Model file for the job. Use its own axes, mm. Give positions to 0.01 mm unless a question says otherwise; leave off trailing zeros. Loops run counter-clockwise (first coordinate to the right, second up) from the corner with the lowest first, then second, coordinate; pieces in that order, holes last. Notation, with made-up numbers: M 17.5,0 L 49.5,0 A22 cw 49.5,29 Z; hole C 74.25,-40 d5. An arc over 180 degrees is marked long. Answer in a Markdown table with one row per item.
```python
from build123d import *

# Parameters (mm, degrees)
SKETCH2_W                            = 300
SKETCH2_H                            = 150
BOSS_EXTRUDE1_DEPTH                  = 1.52
F_4_0_4_DIAMETER_HOLE1_D             = 4
MIRROR1_AT_THE_SECOND_PLANE_COPY_1_D = 4
F_11_0_11_DIAMETER_HOLE4_D           = 11
F_11_0_11_DIAMETER_HOLE2_D           = 11
F_11_0_11_DIAMETER_HOLE3_D           = 11


with BuildPart() as part:
    # Sketch2 → Boss-Extrude1 (new body)
    with BuildSketch(Plane.YZ):
        Rectangle(SKETCH2_W, SKETCH2_H)
    extrude(amount=BOSS_EXTRUDE1_DEPTH)

    # Ø4.0 (4) Diameter Hole1 (through all)
    with Locations(Plane.YZ.offset(1.52)):
        with Locations((-137.3, 62.3)):
            f_4_0_4_diameter_hole1 = Hole(F_4_0_4_DIAMETER_HOLE1_D / 2)

    # Mirror1: Ø4.0 (4) Diameter Hole1 across plane
    add(f_4_0_4_diameter_hole1.mirror(Plane.ZX), mode=Mode.SUBTRACT)

    # Mirror1 at the second plane: Ø4.0 (4) Diameter Hole1 across plane
    add(f_4_0_4_diameter_hole1.mirror(Plane.XY), mode=Mode.SUBTRACT)

    # Mirror1 at the second plane copy 1 (through all)
    with Locations(Plane(origin=(1.52, 0, 0), x_dir=(0, -1, 0), z_dir=(1, 0, 0))):
        with Locations((-137.3, 62.3)):
            Hole(MIRROR1_AT_THE_SECOND_PLANE_COPY_1_D / 2)

    # Ø11.0 (11) Diameter Hole4 (through all)
    with Locations(Plane.YZ.offset(1.52)):
        with Locations((-95, 30), (-45, 30)):
            f_11_0_11_diameter_hole4 = Hole(F_11_0_11_DIAMETER_HOLE4_D / 2)

    # Mirror2: Ø11.0 (11) Diameter Hole4 across plane
    add(f_11_0_11_diameter_hole4.mirror(Plane.XY), mode=Mode.SUBTRACT)

    # Ø11.0 (11) Diameter Hole2 (through all)
    with Locations(Plane.YZ.offset(1.52)):
        with Locations((0, 20), (35, 20), (70, 20)):
            f_11_0_11_diameter_hole2 = Hole(F_11_0_11_DIAMETER_HOLE2_D / 2)

    # Mirror3: Ø11.0 (11) Diameter Hole2 across plane
    add(f_11_0_11_diameter_hole2.mirror(Plane.XY), mode=Mode.SUBTRACT)

    # Ø11.0 (11) Diameter Hole3 (through all)
    with Locations(Plane.YZ.offset(1.52)):
        with Locations((105, 0)):
            Hole(F_11_0_11_DIAMETER_HOLE3_D / 2)


solid = part.part
```
(1) Saw through at B-B, the plane z = 20. Give the cut face in (x, y), and give its area (3 significant figures).
Established:
| item | result |
|---|---|
| outline | M 0,-150 L 1.52,-150 L 1.52,-5.5 L 0,-5.5 Z; M 0,5.5 L 1.52,5.5 L 1.52,29.5 L 0,29.5 Z; M 0,40.5 L 1.52,40.5 L 1.52,64.5 L 0,64.5 Z; M 0,75.5 L 1.52,75.5 L 1.52,150 L 0,150 Z |
| area | 406 mm2 |
(2) Saw through at C-C, the plane x = 0.3. Count the separate pieces of the cut face and the enclosed holes in it, and give its area (3 significant figures).
Established:
| item | result |
|---|---|
| separate pieces | 1 |
| enclosed holes | 15 |
| area | 43,900 mm2 |
(3) Wall check: L1, parallel to Z at x = 0.45, y = -45; L2, parallel to Z at x = 0.85, y = 0; L3, parallel to Y at x = 1.1, z = -29. Give the ranges that are in metal, low to high.
Established:
| item | result |
|---|---|
| L1 | z = -75 to -35.5, -24.5 to 24.5, 35.5 to 75 |
| L2 | z = -75 to -25.5, -14.5 to 14.5, 25.5 to 75 |
| L3 | y = -150 to -100.41, -89.59 to -50.41, -39.59 to 150 |
(4) Flat gauge pin, fed straight in: P1, Ø3.5, axis at y = 137.3, z = -62.3, coming from the +X side. Where does the tip first touch, or does it go through?
Established:
| item | result |
|---|---|
| P1 | passes through |
(5) Mould opens along Y. For faces 1 (the cylindrical face through (0.749, 35.716, -25.453)), 2 (the flat face through (0, -2, 1)), 3 (the cylindrical face through (0.749, 75.495, -20.242)) say: pulls with the +Y half, pulls with the -Y half, needs draft (parallel to the pull), parting line crosses it, or undercut.
Established:
| item | result |
|---|---|
| face 1 | undercut |
| face 2 | needs draft |
| face 3 | undercut |
(6) Saw through at A-A, the plane y = 0. Give the cut face in (x, z), and give its area (3 significant figures).
Established:
| item | result |
|---|---|
| outline | M 0,-75 L 1.52,-75 L 1.52,-25.5 L 0,-25.5 Z; M 0,-14.5 L 1.52,-14.5 L 1.52,14.5 L 0,14.5 Z; M 0,25.5 L 1.52,25.5 L 1.52,75 L 0,75 Z |
| area | 195 mm2 |
